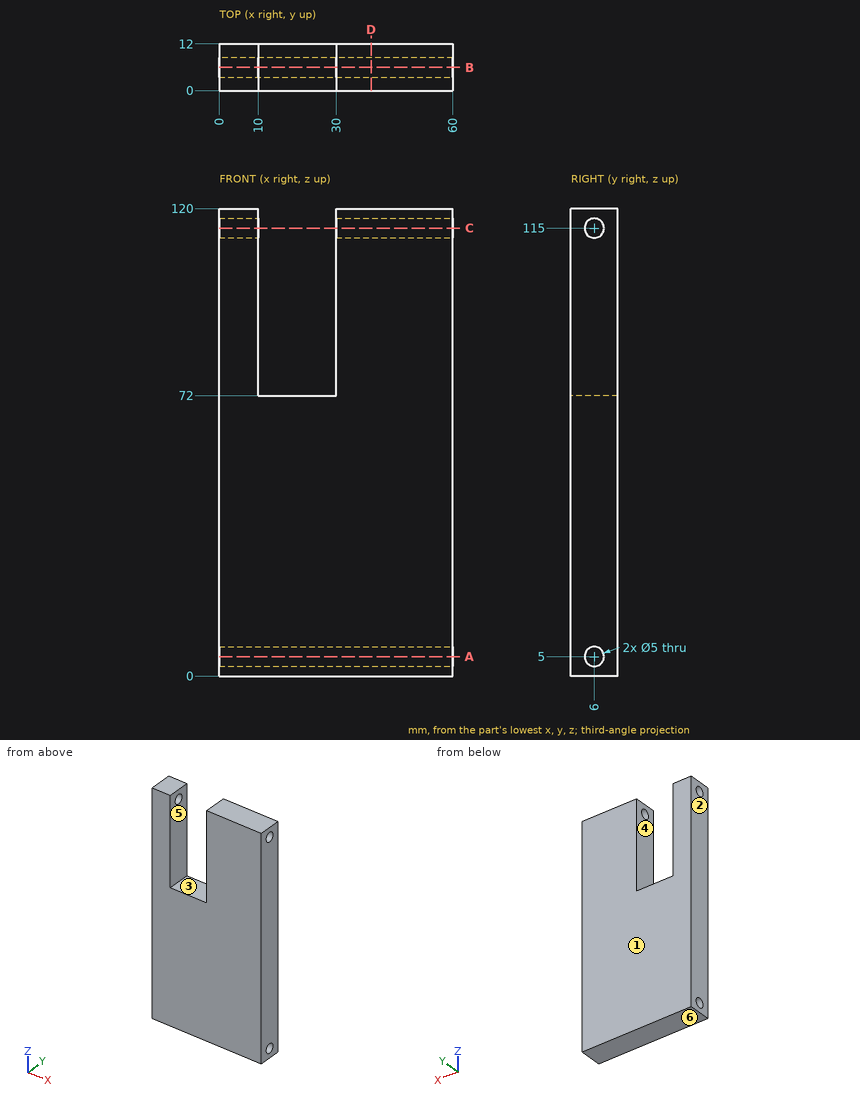
Check sheet for the drawn part. Datum: minimum x, y, z corner. Units: mm. A direction names the side the tool comes from. Round coordinates to 2 decimals unless told otherwise and drop trailing zeros. Order: outer loops, then holes, each group sorted by start corner. A loop starts at its lowest first (then second) coordinate and runs counter-clockwise, first axis right, second up. Notation, with made-up numbers: (63.5, 7) - (89.5, 7) arc R28 cw to (89.5, 25) - close; hole circle Ø2 at (38, 85). An arc over 180 degrees is marked (long way). Use a Markdown table: item, result. Add a question column.
(1) Depth check by flat-ended pin: pin 1 (3 mm diameter, centred on x = 16, y = 4, fed in from +Z). Enter the tip coordinate at first touch or a pass-through.
(2) Sectioned sample at B-B, the plane y = 6. Enter the section's corners in (x, z), and give its area (3 significant figures).
(3) Material ranges on line 1 along Z through (x, y) = (38, 6); line 2 along X through (y, z) = (3, 104); line 3 along Z through (x, y) = (5, 4), recorded low to high. Write a range as [from, to].
(4) Release check for a two-part mould opening along X. For the marked faces 1, 2, 3 and 4 record: pulls with the +X half, pulls with the -X half, needs draft (parallel to the pull), parting line crosses it, or undercut.
(5) Tool access check on the marked faces 5 and 6. Record the directions out of +Z, -Z, +X, -X, +Y, -Y that give a thin tool (end or side, any length) a straight path to the whole face; none if there is none.
(6) Sectioned sample at C-C, the plane z = 115. Enter the section's corners in (x, y), and give its area (3 significant figures).
(7) Sectioned sample at A-A, the plane z = 5. Enter the section's corners in (x, y).
(8) Sectioned sample at D-D, the plane x = 39. Enter the section's corners in (y, z).
Answers below:
| question | item | result |
|---|---|---|
| 1 | pin 1 | z = 72 |
| 2 | outline | (0, 0) - (60, 0) - (60, 2.5) - (0, 2.5) - close; (0, 7.5) - (60, 7.5) - (60, 112.5) - (30, 112.5) - (30, 72) - (10, 72) - (10, 112.5) - (0, 112.5) - close; (0, 117.5) - (10, 117.5) - (10, 120) - (0, 120) - close; (30, 117.5) - (60, 117.5) - (60, 120) - (30, 120) - close |
| 2 | area | 5,740 mm² |
| 3 | line 1 | [0, 2.5], [7.5, 112.5], [117.5, 120] |
| 3 | line 2 | [0, 10], [30, 60] |
| 3 | line 3 | [0, 3.5], [6.5, 113.5], [116.5, 120] |
| 4 | face 1 | needs draft |
| 4 | face 2 | pulls with the -X half |
| 4 | face 3 | undercut |
| 4 | face 4 | undercut |
| 5 | face 5 | +Z, +Y, -Y |
| 5 | face 6 | -Z, +X, -X, +Y, -Y |
| 6 | outline | (0, 0) - (10, 0) - (10, 3.5) - (0, 3.5) - close; (0, 8.5) - (10, 8.5) - (10, 12) - (0, 12) - close; (30, 0) - (60, 0) - (60, 3.5) - (30, 3.5) - close; (30, 8.5) - (60, 8.5) - (60, 12) - (30, 12) - close |
| 6 | area | 280 mm² |
| 7 | outline | (0, 0) - (60, 0) - (60, 3.5) - (0, 3.5) - close; (0, 8.5) - (60, 8.5) - (60, 12) - (0, 12) - close |
| 8 | outline | (0, 0) - (12, 0) - (12, 120) - (0, 120) - close; hole circle Ø5 at (6, 5); hole circle Ø5 at (6, 115) |
